```python
from build123d import *

# Parameters (mm, degrees)
RESSALTO_EXTRUS_O1_DEPTH = 15
ESBO_O2_R                = 5
CORTE_EXTRUS_O1_DEPTH    = 21


with BuildPart() as part:
    # Esboço1 → Ressalto-extrusão1 (new body)
    with BuildSketch(Plane.XY):
        Polygon((0, 0), (20, 0), (20, 3), (5, 3), (5, 50), (0, 50), align=None)
    extrude(amount=RESSALTO_EXTRUS_O1_DEPTH)

    # Esboço2 → Corte-extrusão1 (cut, through all)
    with BuildSketch(Plane.ZY):
        with Locations((7.5, 42.5)):
            Circle(ESBO_O2_R)
    extrude(amount=-CORTE_EXTRUS_O1_DEPTH, mode=Mode.SUBTRACT)


solid = part.part
```
Geometry check sheet. Reference: the model listing, model coordinates, mm. A direction names the side the tool comes from. Coordinates: 2 decimals unless noted, no trailing zeros. Order: outer loops, then holes, each group sorted by start corner. A loop starts at its lowest first (then second) coordinate and runs counter-clockwise, first axis right, second up. Notation, with made-up numbers: M 75.5,8 L 110.5,8 A24 cw 110.5,47 Z; hole C -32.75,3.25 d10. An arc over 180 degrees is marked long. One line per question, with ' | ' between items. Start each with the question number.
Item 1: Cross-section at A-A on z = 4.5. Enter the section's corners in (x, y), then the cut area to 3 significant figures.
Item 2: Set-up check for faces 5 (the flat face through (4, 21, 0)), 6 (the flat face through (5, 26, 7)): record each of +Z, -Z, +X, -X, +Y, -Y from which the full face is reachable in a straight line by a thin tool's end or side.
Item 3: Gauge pin test, flat ends, axial feed: pin 1 (5 mm diameter, centred on x = 8, y = 40.5, fed in from -Z); pin 2 (3 mm diameter, centred on y = 8.5, z = 11, fed in from +X); pin 3 (6 mm diameter, centred on x = 11, z = 5, fed in from +Y). Record the tip position at first contact, or that the pin passes through.
Item 4: Cross-section at C-C on x = 4.5. Enter the section's corners in (y, z).
Item 5: Cross-section at D-D on z = 13.75. Enter the section's corners in (x, y), then the cut area to 3 significant figures.
Item 6: Draft check along Y on faces 1 (the flat face through (0, 25, 7)), 2 (the flat face through (10, 0, 7)), 3 (the cylindrical face through (2.465, 47.457, 6.849)), 4 (the flat face through (3, 50, 7)). Enter one of: pulls with the +Y half, pulls with the -Y half, needs draft (parallel to the pull), parting line crosses it, or undercut.
Item 7: Material ranges on L1, parallel to Y at x = 2.6, z = 7.5; L2, parallel to X at y = 22, z = 5.5; L3, parallel to Y at x = 16, z = 10.5, recorded low to high. Write a range as [from, to].
Item 8: Cross-section at B-B on y = 42.5. Enter the section's corners in (x, z).
Findings:
1) outline: M 0,0 L 20,0 L 20,3 L 5,3 L 5,38.5 L 0,38.5 Z; M 0,46.5 L 5,46.5 L 5,50 L 0,50 Z | area: 255 mm²
2) face 5: -Z, +X, -X, +Y, -Y | face 6: +Z, -Z, +X, +Y
3) pin 1: passes through | pin 2: stops at x = 5 | pin 3: stops at y = 3
4) outline: M 0,0 L 50,0 L 50,15 L 0,15 Z; hole C 42.5,7.5 d10
5) outline: M 0,0 L 20,0 L 20,3 L 5,3 L 5,50 L 0,50 Z | area: 295 mm²
6) face 1: needs draft | face 2: pulls with the -Y half | face 3: undercut | face 4: pulls with the +Y half
7) L1: y = [0, 37.5], [47.5, 50] | L2: x = [0, 5] | L3: y = [0, 3]
8) outline: M 0,0 L 5,0 L 5,2.5 L 0,2.5 Z; M 0,12.5 L 5,12.5 L 5,15 L 0,15 Z
